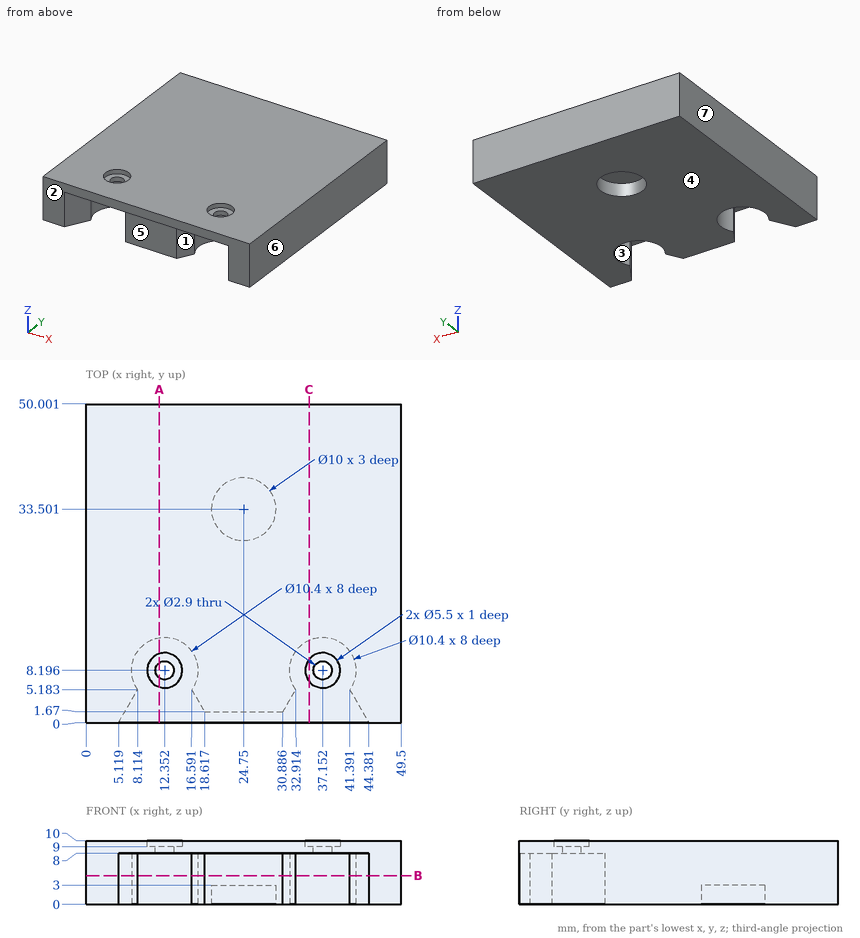
Answer from the drawing. Dimensions are ordinates in mm from the lowest x, y and z of the part. A direction names the side the tool comes from. Coordinates: 2 decimals unless noted, no trailing zeros. Loops run counter-clockwise (first coordinate to the right, second up) from the corner with the lowest first, then second, coordinate; pieces in that order, holes last.
Q1. The part is cut by section A-A on x = 11.5. Write down the section's boundary in (y, z) (1 decimal), and give its area (3 significant figures).
Q2. Consider probe 1 along Y at (x, z) = (30, 2.5); probe 2 along Y at (x, z) = (28, 1.75); probe 3 along Z at (x, y) = (39, 4). Determine where each line is inside the solid, lowest interval first.
Q3. The mould has two halves that part along X. Classify the marked faces 4, 5, 6 and 7: +X half, -X half, draft (parallel to the pull), parting line (faces both ways), or undercut.
Q4. Which of the six approach directions +Z, -Z, +X, -X, +Y, -Y give full straight-line access (tool end or side, diameter ignored) to the marked faces 1, 2 and 3?
Q5. The part is cut by section B-B on z = 4.5. Write down the section's boundary in (x, y) (1 decimal).
Q6. Each of these flat-tipped pins is pushed along its axis until it touches: pin 1 Ø9.5 at (x, y) = (12.35, 8.2) entering from -Z; pin 2 Ø1.6 at (x, y) = (37, 7) entering from +Z; pin 3 Ø3 at (x, y) = (23, 33) entering from -Z. Where does it stop, or does it pass through?
Q7. The part is cut by section C-C on x = 35. Write down the section's boundary in (y, z) (1 decimal).
Results below:
1. outline: (0, 8) - (7, 8) - (7, 9) - (5.6, 9) - (5.6, 10) - (0, 10) - close; (9.4, 8) - (13.3, 8) - (13.3, 0) - (50, 0) - (50, 10) - (10.8, 10) - (10.8, 9) - (9.4, 9) - close
1. area: 386 mm2
2. probe 1: y = 1.67 to 50
2. probe 2: y = 1.67 to 29.7, 37.3 to 50
2. probe 3: z = 8 to 10
3. face 4: draft
3. face 5: undercut
3. face 6: +X half
3. face 7: -X half
4. face 1: -Z, -Y
4. face 2: +Z, -Z, +X, -X, -Y
4. face 3: -Z
5. outline: (0, 0) - (5.1, 0) - (8.1, 5.2) arc R5.2 cw (long way) to (16.6, 5.2) - (18.6, 1.7) - (30.9, 1.7) - (32.9, 5.2) arc R5.2 cw (long way) to (41.4, 5.2) - (44.4, 0) - (49.5, 0) - (49.5, 50) - (0, 50) - close
6. pin 1: stops at z = 8
6. pin 2: stops at z = 9
6. pin 3: stops at z = 3
7. outline: (0, 8) - (12.9, 8) - (12.9, 0) - (50, 0) - (50, 10) - (9.9, 10) - (9.9, 9) - (6.5, 9) - (6.5, 10) - (0, 10) - close
